```python
from build123d import *

# Parameters (mm, degrees)
SKETCH1_R           = 3
SKETCH1_R_2         = 9.45
BOSS_EXTRUDE1_DEPTH = 30.6
CUT_EXTRUDE1_DEPTH  = 26.1


with BuildPart() as part:
    # Sketch1 → Boss-Extrude1 (new body)
    with BuildSketch(Plane.XY):
        with BuildLine():
            ThreePointArc((74.571121214, -32.760854905), (98.6, 0), (74.571121214, 32.760854905))
            Line((74.571121214, 32.760854905), (16.117374778, 51.171796238))
            ThreePointArc((16.117374778, 51.171796238), (-53.65, 0), (16.117374778, -51.171796238))
            Line((16.117374778, -51.171796238), (74.571121214, -32.760854905))
        make_face()
        with BuildLine():
            Line((63.4, 10.4), (65.5, 10.4))
            ThreePointArc((65.5, 10.4), (75.9, 0), (65.5, -10.4))
            Line((65.5, -10.4), (63.4, -10.4))
            ThreePointArc((63.4, -10.4), (53, 0), (63.4, 10.4))
        make_face(mode=Mode.SUBTRACT)
        with Locations((30.05, 0)):
            Circle(SKETCH1_R, mode=Mode.SUBTRACT)
        with BuildLine():
            Line((56.551094978, -17.45), (54.701094978, -17.45))
            ThreePointArc((54.701094978, -17.45), (52.701094978, -15.45), (54.701094978, -13.45))
            Line((54.701094978, -13.45), (56.551094978, -13.45))
            ThreePointArc((56.551094978, -13.45), (58.551094978, -15.45), (56.551094978, -17.45))
        make_face(mode=Mode.SUBTRACT)
        with BuildLine():
            Line((87.601094978, -17.45), (85.751094978, -17.45))
            ThreePointArc((85.751094978, -17.45), (83.751094978, -15.45), (85.751094978, -13.45))
            Line((85.751094978, -13.45), (87.601094978, -13.45))
            ThreePointArc((87.601094978, -13.45), (89.601094978, -15.45), (87.601094978, -17.45))
        make_face(mode=Mode.SUBTRACT)
        with BuildLine():
            ThreePointArc((54.701094978, 13.45), (52.701094978, 15.45), (54.701094978, 17.45))
            Line((54.701094978, 17.45), (56.551094978, 17.45))
            ThreePointArc((56.551094978, 17.45), (58.551094978, 15.45), (56.551094978, 13.45))
            Line((56.551094978, 13.45), (54.701094978, 13.45))
        make_face(mode=Mode.SUBTRACT)
        with BuildLine():
            ThreePointArc((85.751094978, 13.45), (83.751094978, 15.45), (85.751094978, 17.45))
            Line((85.751094978, 17.45), (87.601094978, 17.45))
            ThreePointArc((87.601094978, 17.45), (89.601094978, 15.45), (87.601094978, 13.45))
            Line((87.601094978, 13.45), (85.751094978, 13.45))
        make_face(mode=Mode.SUBTRACT)
        Circle(SKETCH1_R_2, mode=Mode.SUBTRACT)
        with Locations((0, 30.05)):
            Circle(SKETCH1_R, mode=Mode.SUBTRACT)
        with Locations((0, -30.05)):
            Circle(SKETCH1_R, mode=Mode.SUBTRACT)
        with Locations((-30.05, 0)):
            Circle(SKETCH1_R, mode=Mode.SUBTRACT)
    extrude(amount=BOSS_EXTRUDE1_DEPTH)

    # Sketch2 → Cut-Extrude1 (cut)
    with BuildSketch(Plane.XY.offset(30.6)):
        with BuildLine():
            Line((74.180579048, 31.520904576), (15.726832612, 49.93184591))
            ThreePointArc((15.726832612, 49.93184591), (-52.35, 0), (15.726832612, -49.93184591))
            Line((15.726832612, -49.93184591), (74.180579048, -31.520904576))
            ThreePointArc((74.180579048, -31.520904576), (97.3, 0), (74.180579048, 31.520904576))
        make_face()
    extrude(amount=-CUT_EXTRUDE1_DEPTH, mode=Mode.SUBTRACT)


solid = part.part
```
Build history of the part. All positions in model axes, mm. A direction names the side the tool comes from. Round coordinates to 2 decimals unless told otherwise and drop trailing zeros. Write each loop counter-clockwise with the first axis right and the second up, starting at its lowest first coordinate (ties: lowest second). Pieces come first, ordered by that corner, then holes.
1) Band-saw the part on B-B, the plane z = 18. List the corners of the cut face in (x, y), and give its area (3 significant figures).
2) Band-saw the part on A-A, the plane x = 0. List the corners of the cut face in (y, z), and give its area (3 significant figures).
3) Band-saw the part on C-C, the plane y = -15.45. List the corners of the cut face in (x, z).
4) 3-axis set-ups, long thin cutter, end or side, ignore diameter. For faces 1 (the cylindrical face through (52.7, -15.5, 2.2)), 2 (the flat face through (45.75, 41.84, 15.09)), 3 (the flat face through (44.545, -40.855, 17.733)): which of +Z, -Z, +X, -X, +Y, -Y reach the whole face in a straight line?
5) Pin check, flat tips, straight feed: pin 1 (1.5 mm diameter, centred on x = 56, z = 1.5, fed in from -Y); pin 2 (3 mm diameter, centred on x = -35.5, y = -30, fed in from +Z); pin 3 (2 mm diameter, centred on x = 55, z = 3, fed in from +Y). Stop position of each tip, or through.
6) Mould opens along X. For faces 4 (the cylindrical face through (98.595, -0.609, 15.086)), 5 (the flat face through (45.36, 40.6, 17.73)), 6 (the flat face through (28, -47, 30.6)), 7 (the cylindrical face through (-53.63, 1.41, 15.09)) say: +X half, -X half, draft (parallel to the pull), parting line (faces both ways), or undercut.
7) Band-saw the part on D-D, the plane x = 37.5. List the corners of the cut face in (y, z).
8) Drill centre lines: probe 1 along Y at (x, z) = (0, 3.65); probe 2 along Y at (x, z) = (0, 16); probe 3 along Z at (x, y) = (36.5, 36). Where is each one in solid material? Low to high.
Ans:
1. outline: (16.12, -51.17) - (74.57, -32.76) arc R34.35 ccw to (74.57, 32.76) - (16.12, 51.17) arc R53.65 ccw (long way) to start; hole (15.73, -49.93) - (74.18, -31.52) arc R33.05 ccw to (74.18, 31.52) - (15.73, 49.93) arc R52.35 ccw (long way) to start
1. area: 529 mm2
2. outline: (-53.65, 0) - (-33.05, 0) - (-33.05, 4.5) - (-52.35, 4.5) - (-52.35, 30.6) - (-53.65, 30.6) - close; (-27.05, 0) - (-9.45, 0) - (-9.45, 4.5) - (-27.05, 4.5) - close; (9.45, 0) - (27.05, 0) - (27.05, 4.5) - (9.45, 4.5) - close; (33.05, 0) - (53.65, 0) - (53.65, 30.6) - (52.35, 30.6) - (52.35, 4.5) - (33.05, 4.5) - close
2. area: 412 mm2
3. outline: (-51.38, 0) - (52.7, 0) - (52.7, 4.5) - (-50.02, 4.5) - (-50.02, 30.6) - (-51.38, 30.6) - close; (58.55, 0) - (83.75, 0) - (83.75, 4.5) - (58.55, 4.5) - close; (89.6, 0) - (94.93, 0) - (94.93, 30.6) - (93.47, 30.6) - (93.47, 4.5) - (89.6, 4.5) - close
4. face 1: +Z, -Z
4. face 2: +Z, -Z, +X, +Y
4. face 3: +Z
5. pin 1: stops at y = -38.85
5. pin 2: stops at z = 4.5
5. pin 3: stops at y = 39.24
6. face 4: +X half
6. face 5: undercut
6. face 6: draft
6. face 7: parting line
7. outline: (-44.44, 0) - (44.44, 0) - (44.44, 30.6) - (43.07, 30.6) - (43.07, 4.5) - (-43.07, 4.5) - (-43.07, 30.6) - (-44.44, 30.6) - close
8. probe 1: y = -53.65 to -33.05, -27.05 to -9.45, 9.45 to 27.05, 33.05 to 53.65
8. probe 2: y = -53.65 to -52.35, 52.35 to 53.65
8. probe 3: z = 0 to 4.5
